Solid Edge part; units mm, degrees
sketch "Sketch1" plane through (0, 0, 0) normal (0, -1, 0) x (1, 0, 0)
  line L0 (0, 0) -> (17.5, 0)
  line L1 (17.5, 0) -> (17.5, 20)
  line L2 (17.5, 20) -> (20, 20)
  line L3 (20, 20) -> (20, 28)
  line L4 (20, 28) -> (37.5, 28)
  line L5 (37.5, 28) -> (37.5, 35)
  line L6 (37.5, 35) -> (0, 35)
  dimension "D1" = 17.5
  dimension "D2" = 37.5
  dimension "D3" = 20
revolve "RevolvedProtrusion1" add sketch "Sketch1" angle 360 about axis through (0, 0, 35) along (0, 0, -1)
chamfer "Chamfer1" distance 1 angle 45 1 edges at (-17.5, 0, 0)
hole "Hole_1" at (0, 0, 35) direction (0, 0, -1) diameter 5 end up to next
chamfer "Chamfer_2" distance 1 angle 45 1 edges at (-2.5, 0, 0)
hole "Hole_2" at (20, 20, 35) direction (0, 0, -1) diameter 4.8 end up to next
hole "Hole1" at (20, -20, 35) direction (0, 0, -1) diameter 4.8 end up to next
hole "Hole2" at (-20, -20, 35) direction (0, 0, -1) diameter 4.8 end up to next
hole "Hole3" at (-20, 20, 35) direction (0, 0, -1) diameter 4.8 end up to next
hole "Hole_6" at (0, -30, 28) direction (0, 0, 1) diameter 4.8 end up to next counterbore diameter 8 counterbore depth 4.8
hole "Hole4" at (30, 0, 28) direction (0, 0, 1) diameter 4.8 end up to next counterbore diameter 8 counterbore depth 4.8
hole "Hole5" at (0, 30, 28) direction (0, 0, 1) diameter 4.8 end up to next counterbore diameter 8 counterbore depth 4.8
hole "Hole6" at (-30, 0, 28) direction (0, 0, 1) diameter 4.8 end up to next counterbore diameter 8 counterbore depth 4.8
properties material "Polyethylene, low density"
Source: CAD feature listing. Evaluate the final solid. Frame: model axes, mm. A direction names the side the tool comes from. Round coordinates to 2 decimals unless told otherwise and drop trailing zeros. Loops run counter-clockwise (first coordinate to the right, second up) from the corner with the lowest first, then second, coordinate; pieces in that order, holes last. Notation, with made-up numbers: (16.5, 85) - (60.5, 85) arc R28 cw to (60.5, 115) - close; hole circle Ø8 at (1, 24.5). An arc over 180 degrees is marked (long way). Use CSV: the item, a comma, the result in double quotes.
Q1. Section query D-D, the plane z = 13. Output: boundary loops of the cut face in (x, y), then the cut area to 3 significant figures.
Reported:
outline,"circle Ø35 at (0, 0); hole circle Ø5 at (0, 0)"
area,"942 mm^2"
Q2. Section query C-C, the plane y = 0. Give the number of separate pieces and of enclosed holes in the cut face, then the cut area to 3 significant figures.
Reported:
separate pieces,"4"
enclosed holes,"0"
area,"1,270 mm^2"
Q3. Reachability of faces 5 (the cylindrical face through (-2.44, 0.54, 18.24)), 6 (the flat face through (16, 16, 28)) from +Z, -Z, +X, -X, +Y, -Y: full face, straight path, thin tool, end or side. Return the list, or none.
Reported:
face 5,"+Z, -Z"
face 6,"-Z"
Q4. Section query B-B, the plane y = -21.5. Output: boundary loops of the cut face in (x, z).
Reported:
outline,"(-30.72, 28) - (-21.87, 28) - (-21.87, 35) - (-30.72, 35) - close; (-18.13, 28) - (18.13, 28) - (18.13, 35) - (-18.13, 35) - close; (21.87, 28) - (30.72, 28) - (30.72, 35) - (21.87, 35) - close"
Q5. Ray query, line 1 along Y through (x, z) = (0, 34); line 2 along X through (y, z) = (0, 29.7). Return the intervals inside material, ascending.
Reported:
line 1,"-37.5 to -32.4, -27.6 to -2.5, 2.5 to 27.6, 32.4 to 37.5"
line 2,"-37.5 to -34, -26 to -2.5, 2.5 to 26, 34 to 37.5"
Q6. Pin query (flat end, axial travel): pin 1 Ø10 at (x, y) = (-9, 0) entering from -Z; pin 2 Ø12 at (y, z) = (7, 18) entering from -X; pin 3 Ø8 at (x, z) = (-25, 28) entering from -Y; pin 4 Ø6.5 at (x, y) = (0.5, -29.5) entering from -Z. Return the tip coordinate at first contact, or that it passes through.
Reported:
pin 1,"z = 0"
pin 2,"x = -19.95"
pin 3,"y = -31.07"
pin 4,"z = 32.8"
Q7. Section query A-A, the plane x = -21. Output: boundary loops of the cut face in (y, z).
Reported:
outline,"(-31.07, 28) - (-22.18, 28) - (-22.18, 35) - (-31.07, 35) - close; (-17.82, 28) - (17.82, 28) - (17.82, 35) - (-17.82, 35) - close; (22.18, 28) - (31.07, 28) - (31.07, 35) - (22.18, 35) - close"
Q8. Mould query, pull axis X, two halves, no side actions, for faces 1 (the flat face through (2, 32, 32.8)), 2 (the cylindrical face through (2.4, 26.8, 30.4)), 3 (the cylindrical face through (-13.887, -10.648, 10.633)), 4 (the flat face through (-1, 8, 35)). Classes: pulls with the +X half, pulls with the -X half, needs draft (parallel to the pull), parting line crosses it, or undercut.
Reported:
face 1,"undercut"
face 2,"undercut"
face 3,"parting line crosses it"
face 4,"needs draft"
